from build123d import *

# Parameters (mm, degrees)
SKETCH236_W      = 25
SKETCH236_H      = 9
PAD097_DEPTH     = 20
SKETCH237_W      = 18
SKETCH237_H      = 20
PAD098_DEPTH     = 2.5
SKETCH238_R      = 1.75
POCKET034_DEPTH  = 11
CHAMFER030_SIZE  = 2
SKETCH239_R      = 2.25
POCKET035_DEPTH  = 8
CHAMFER031_SIZE2 = 12
CHAMFER031_SIZE  = 15
SKETCH240_W      = 18
SKETCH240_H      = 2.5
PAD099_DEPTH     = 1
FILLET025_R      = 5


with BuildPart() as body044:
    # Sketch236 → Pad097 (new body)
    with BuildSketch(Plane.XZ):
        with Locations((12.5, 0)):
            Rectangle(SKETCH236_W, SKETCH236_H)
    extrude(amount=-PAD097_DEPTH)

    # Sketch237 (on Face2 of Pad097) → Pad098 (join)
    with BuildSketch(Plane(origin=(0, 0, -4.5), x_dir=(1, 0, 0), z_dir=(0, 0, -1))):
        with Locations((16, -10)):
            Rectangle(SKETCH237_W, SKETCH237_H)
    extrude(amount=PAD098_DEPTH)

    # Sketch238 (on Face3 of Pad098) → Pocket034 (cut)
    with BuildSketch(Plane(origin=(0, 0, -4.5), x_dir=(1, 0, 0), z_dir=(0, 0, -1))):
        with Locations((4.5, -5)):
            Circle(SKETCH238_R)
        with Locations((4.5, -15)):
            Circle(SKETCH238_R)
    extrude(amount=-POCKET034_DEPTH, mode=Mode.SUBTRACT)

    # Chamfer030
    chamfer030_edges = [body044.edges().sort_by_distance(p)[0] for p in [
        (2.75, 15, 4.5),
        (2.75, 5, 4.5),
    ]]
    chamfer(chamfer030_edges, length=CHAMFER030_SIZE)

    # Sketch239 (on Face4 of Chamfer030) → Pocket035 (cut)
    with BuildSketch(Plane.XZ):
        with Locations((20, 0)):
            Circle(SKETCH239_R)
    extrude(amount=-POCKET035_DEPTH, mode=Mode.SUBTRACT)

    # Chamfer031
    chamfer031_edges = [body044.edges().sort_by_distance(p)[0] for p in [
        (25, 20, -1.25),
    ]]
    chamfer031_side = body044.faces().sort_by_distance((13.083333, 20, -0.958333))[0]
    chamfer(chamfer031_edges, length=CHAMFER031_SIZE, length2=CHAMFER031_SIZE2, reference=chamfer031_side)

    # Sketch240 (on Face6 of Chamfer031) → Pad099 (join)
    with BuildSketch(Plane.XZ):
        with Locations((16, -5.75)):
            Rectangle(SKETCH240_W, SKETCH240_H)
    extrude(amount=PAD099_DEPTH)

    # Fillet025
    fillet025_edges = [body044.edges().sort_by_distance(p)[0] for p in [
        (25, 8, -1.25),
        (10, 20, -1.25),
    ]]
    fillet(fillet025_edges, radius=FILLET025_R)


with BuildPart() as body044_1:
    # Body044 placement: moved
    add(body044.part.moved(Location((10, 0, 0))))


with BuildPart() as part_mirroring002:
    # Part__Mirroring002: instance of Body044
    add(body044_1.part.mirror(Plane(origin=(0, 0, 0), x_dir=(0, -1, 0), z_dir=(1, 0, 0))))


with BuildPart() as part_mirroring002_1:
    # Part__Mirroring002 placement: moved
    add(part_mirroring002.part.moved(Location((-20, 0, 0))))


solid = part_mirroring002_1.part
Input: part model. Units: mm. Frame: model coordinates. A direction names the side the tool comes from. Round coordinates to 2 decimals unless told otherwise and drop trailing zeros. Order: outer loops, then holes, each group sorted by start corner. A loop starts at its lowest first (then second) coordinate and runs counter-clockwise, first axis right, second up. Notation, with made-up numbers: (74, 63.25) - (81, 63.25) arc R38 cw to (81, 102.25) - close; hole circle Ø9 at (31, -13). An arc over 180 degrees is marked (long way). Answer as a JSON object with one key per item and string values. Group by question number.
(1) Cut plane A-A (y = 5). Return loops of the section in (x, z).
(2) Material intervals for probe 1 along Y at (x, z) = (-34.5, -0.5); probe 2 along Z at (x, y) = (-50, 5); probe 3 along X at (y, z) = (5, 0.25), sorted ascending. Write a range as from..to.
(3) Cut plane B-B (x = -34.5). Return loops of the section in (y, z), then the cut area to 3 significant figures.
(4) Draft query along Y for faces 4 (the face through (-32.75, 4.92, -1.05)), 5 (the face through (-33, 10, -4.5)), 6 (the face through (-34, 20, 0)). Return one class per face: released by +Y, released by -Y, zero draft, split by the parting line, or undercut.
(5) Cut plane D-D (z = 0). Return loops of the section in (x, y), then the cut area to 3 significant figures.
(6) Reachability of faces 1 (the face through (-42, 0, 0)), 2 (the face through (-50, 8, 0)), 3 (the face through (-37, 10, -6)) from +Z, -Z, +X, -X, +Y, -Y: full face, straight path, thin tool, end or side. Return the list, or none.
(7) Pin query (flat end, axial travel): P1, Ø2, axis at x = -34, y = 7, coming from the -Z side; P2, Ø5, axis at x = -50, z = 0, coming from the -Y side; P3, Ø1.3, axis at x = -49, z = -1, coming from the -Y side. Return the tip coordinate at first contact, or that it passes through.
(8) Cut plane C-C (y = 15). Return loops of the section in (x, z).
Here are the results:
{
 "1": {"outline": "(-55, -7) - (-37, -7) - (-37, -4.5) - (-36.25, -4.5) - (-36.25, 2.5) - (-38.25, 4.5) - (-55, 4.5) - close; (-32.75, -4.5) - (-30, -4.5) - (-30, 4.5) - (-30.75, 4.5) - (-32.75, 2.5) - close; hole circle Ø4.5 at (-50, 0)"},
 "2": {"probe 1": "y = 0..3.25, 6.75..13.25, 16.75..20", "probe 2": "z = -7..-2.25, 2.25..4.5", "probe 3": "x = -55..-52.24, -47.76..-36.25, -32.75..-30"},
 "3": {"outline": "(0, -4.5) - (3.25, -4.5) - (3.25, 2.5) - (1.25, 4.5) - (0, 4.5) - close; (6.75, -4.5) - (13.25, -4.5) - (13.25, 2.5) - (11.25, 4.5) - (8.75, 4.5) - (6.75, 2.5) - close; (16.75, -4.5) - (20, -4.5) - (20, 4.5) - (18.75, 4.5) - (16.75, 2.5) - close", "area": "109 mm^2"},
 "4": {"face 4": "undercut", "face 5": "zero draft", "face 6": "released by +Y"},
 "5": {"outline": "(-55, 0) - (-52.25, 0) - (-52.25, 8) - (-47.75, 8) - (-47.75, 0) - (-30, 0) - (-30, 20) - (-38.25, 20) arc R5 ccw to (-41.37, 18.9) - (-53.12, 9.5) arc R5 ccw to (-55, 5.6) - close; hole circle Ø3.5 at (-34.5, 5); hole circle Ø3.5 at (-34.5, 15)", "area": "354 mm^2"},
 "6": {"face 1": "+Z, +X, -X, -Y", "face 2": "-Y", "face 3": "-Z, +X, +Y, -Y"},
 "7": {"P1": "stops at z = -4.5", "P2": "stops at y = 0", "P3": "stops at y = 8"},
 "8": {"outline": "(-46.25, -7) - (-37, -7) - (-37, -4.5) - (-36.25, -4.5) - (-36.25, 2.5) - (-38.25, 4.5) - (-46.25, 4.5) - close; (-32.75, -4.5) - (-30, -4.5) - (-30, 4.5) - (-30.75, 4.5) - (-32.75, 2.5) - close"}
}
